Source: CAD feature listing. Evaluate the final solid. Frame: model axes, mm. Face numbers are marked on the shaded views. A direction names the side the tool comes from. Coordinates: 2 decimals unless noted, no trailing zeros. Write each loop counter-clockwise with the first axis right and the second up, starting at its lowest first coordinate (ties: lowest second). Pieces come first, ordered by that corner, then holes. Notation, with made-up numbers: (66.25, 18.5) -> (113.25, 18.5) arc R9 cw to (113.25, 26.5) -> close; hole circle Ø7 at (80, 48). An arc over 180 degrees is marked (long way). Write item = value, one per line.
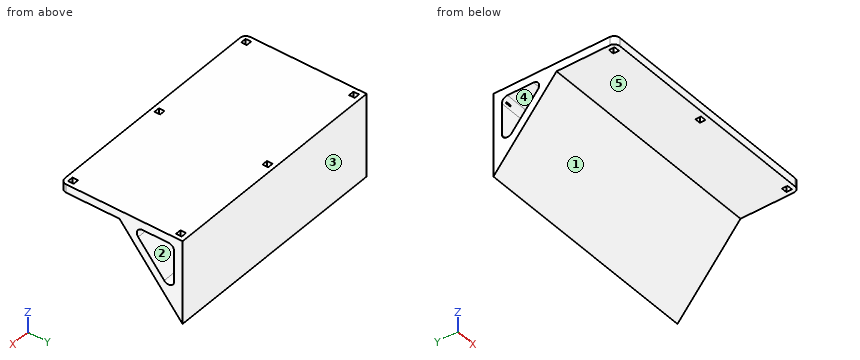
from build123d import *

# Parameters (mm, degrees)
F1_DEPTH = 84
F2_R     = 2
F3_R     = 2
F4_W     = 2
F4_H     = 2
F5_DEPTH = 4


# Not quite as in the source:
# - a feature names something its author has since deleted; it is built from what else it names


with BuildPart() as f1:
    # F0 (on Right) → F1 (new body)
    with BuildSketch(Plane.YZ):
        Polygon((0, 3), (0, 0), (21, 0), (43.497566339, -26.8115555092), (43.497566339, 3), (21, 3), align=None)
        Polygon((40.497566339, -18.5691232508), (24.916221868, 0), (40.497566339, 0), align=None, mode=Mode.SUBTRACT)
    extrude(amount=-F1_DEPTH)

    # F2
    f2_edges = [f1.edges().sort_by_distance(p)[0] for p in [
        (0, 0, 1.5),
        (-84, 0, 1.5),
    ]]
    fillet(f2_edges, radius=F2_R)

    # F3
    f3_edges = [f1.edges().sort_by_distance(p)[0] for p in [
        (-42, 40.497566, 0),
        (-42, 40.497566, -18.569123),
        (-42, 24.916222, 0),
    ]]
    fillet(f3_edges, radius=F3_R)

    # F4 (on face) → F5 (cut)
    with BuildSketch(Plane.XY.offset(3)):
        with Locations((-42, 40.997566339)):
            Rectangle(F4_W, F4_H)
        with Locations((-2.5, 40.997566339)):
            Rectangle(F4_W, F4_H)
        with Locations((-2.5, 2.5)):
            Rectangle(F4_W, F4_H)
        with Locations((-42, 2.4999999997)):
            Rectangle(F4_W, F4_H)
        with Locations((-81.5, 2.5)):
            Rectangle(F4_W, F4_H)
        with Locations((-81.5, 40.997566339)):
            Rectangle(F4_W, F4_H)
    extrude(amount=-F5_DEPTH, mode=Mode.SUBTRACT)


solid = f1.part
1) Reachability of the marked faces 1 and 2 from +Z, -Z, +X, -X, +Y, -Y: full face, straight path, thin tool, end or side. Return the list, or none.
Answer block:
face_1 = -Z, +X, -X, -Y
face_2 = +X, -X
2) Cut plane C-C, the plane z = -11.25. Output: boundary loops of the cut face in (x, y), and give its area (3 significant figures).
Answer block:
outline = (-84, 30.44) -> (0, 30.44) -> (0, 34.36) -> (-84, 34.36) -> close; (-84, 40.5) -> (0, 40.5) -> (0, 43.5) -> (-84, 43.5) -> close
area = 581 mm2
3) Cut plane A-A, the plane x = -20.5. Output: boundary loops of the cut face in (y, z).
Answer block:
outline = (0, 0) -> (21, 0) -> (43.5, -26.81) -> (43.5, 3) -> (0, 3) -> close; hole (27.67, -3.29) -> (36.97, -14.36) arc R2 ccw to (40.5, -13.07) -> (40.5, -2) arc R2 ccw to (38.5, 0) -> (29.21, 0) arc R2 ccw to start
4) First-contact query: pin 1 Ø0.5 at (x, y) = (-81.5, 41) entering from +Z; pin 2 Ø2 at (x, z) = (-58, -22.5) entering from -Y. Flat tips, straight axial feed; report the tip coordinate or a pass-through.
Answer block:
pin_1 = -1
pin_2 = 39.04
5) Pull-direction query (Z, two-part tool) for the marked faces 3, 4 and 5; classes: +Z half, -Z half, draft (parallel to the pull), parting line (faces both ways), or undercut.
Answer block:
face_3 = draft
face_4 = undercut
face_5 = -Z half
6) Cut plane D-D, the plane z = -23.75. Output: boundary loops of the cut face in (x, y), and give its area (3 significant figures).
Answer block:
outline = (-84, 40.93) -> (0, 40.93) -> (0, 43.5) -> (-84, 43.5) -> close
area = 216 mm2
7) Cut plane B-B, the plane y = 34.5. Output: boundary loops of the cut face in (x, z).
Answer block:
outline = (-84, -16.09) -> (0, -16.09) -> (0, -11.42) -> (-84, -11.42) -> close; (-84, 0) -> (0, 0) -> (0, 3) -> (-84, 3) -> close
8) Material intervals for probe 1 along Y at (x, z) = (-3.5, -9.5); probe 2 along Z at (x, y) = (-8.5, 12.5); probe 3 along Y at (x, z) = (-40.5, -1.25), sorted ascending. Write a range as [from, to].
Answer block:
probe_1 = [28.97, 32.89], [40.5, 43.5]
probe_2 = [0, 3]
probe_3 = [22.05, 27.35], [40.35, 43.5]
